```python
from build123d import *

# Parameters (mm, degrees)
EXTRUDE_2_DEPTH     = 6
SKETCH_2_R          = 1.55
CUT_EXTRUDE_1_DEPTH = 10
SKETCH_3_R          = 1.55
CUT_EXTRUDE_2_DEPTH = 10
EXTRUDE_4_DEPTH     = 1.5
EXTRUDE_5_DEPTH     = 1.5
SKETCH_5_W          = 6
SKETCH_5_H          = 6
EXTRUDE_6_DEPTH     = 60
CUT_EXTRUDE_3_DEPTH = 60
SKETCH_9_W          = 6
SKETCH_9_H          = 8.845903007
EXTRUDE_7_DEPTH     = 60
SKETCH_10_W         = 5
SKETCH_10_H         = 2
CUT_EXTRUDE_4_DEPTH = 10
SKETCH_11_R         = 1.55
CUT_EXTRUDE_5_DEPTH = 10


with BuildPart() as part:
    # 草图1 → 凸台-拉伸2 (new body)
    with BuildSketch(Plane(origin=(0, 0, 0), x_dir=(1, 0, 0), z_dir=(0, 1, 0))):
        Polygon((-72.757575758, -68.484848485), (-72.757575758, -1.484848485), (71.242424242, -1.484848485), (71.242424242, -68.484848485), (74.242424242, -68.484848485), (74.242424242, -1.484848485), (74.242424242, 1.515151515), (71.242424242, 1.515151515), (-72.757575758, 1.515151515), (-75.757575758, 1.515151515), (-75.757575758, -1.484848485), (-75.757575758, -68.484848485), align=None)
    extrude(amount=EXTRUDE_2_DEPTH)

    # 草图2 → 切除-拉伸1 (cut)
    with BuildSketch(Plane(origin=(-72.757575758, 0, 0), x_dir=(0, 0, -1), z_dir=(1, 0, 0))):
        with Locations((-65.484848485, 3)):
            Circle(SKETCH_2_R)
    extrude(amount=-CUT_EXTRUDE_1_DEPTH, mode=Mode.SUBTRACT)

    # 草图3 → 切除-拉伸2 (cut)
    with BuildSketch(Plane(origin=(74.242424242, 0, 0), x_dir=(0, 0, -1), z_dir=(1, 0, 0))):
        with Locations((-65.484848485, 3)):
            Circle(SKETCH_3_R)
    extrude(amount=-CUT_EXTRUDE_2_DEPTH, mode=Mode.SUBTRACT)

    # 草图6 → 凸台-拉伸4 (add)
    with BuildSketch(Plane(origin=(0, 6, 0), x_dir=(1, 0, 0), z_dir=(0, 1, 0))):
        Polygon((-75.757575758, 1.515151515), (74.242424242, 1.515151515), (74.242424242, -68.484848485), (71.242424242, -68.484848485), (71.242424242, -1.484848485), (-72.757575758, -1.484848485), (-72.757575758, -68.484848485), (-75.757575758, -68.484848485), align=None)
    extrude(amount=EXTRUDE_4_DEPTH)

    # 草图7 → 凸台-拉伸5 (add)
    with BuildSketch(Plane.XZ):
        Polygon((-75.757575758, 68.484848485), (-75.757575758, -1.515151515), (74.242424242, -1.515151515), (74.242424242, 68.484848485), (71.242424242, 68.484848485), (71.242424242, 1.484848485), (-72.757575758, 1.484848485), (-72.757575758, 68.484848485), align=None)
    extrude(amount=EXTRUDE_5_DEPTH)

    # 草图5 → 凸台-拉伸6 (add)
    with BuildSketch(Plane(origin=(0, 0, -1.515151515), x_dir=(-1, 0, 0), z_dir=(0, 0, -1))):
        with Locations((0.757575758, 3)):
            Rectangle(SKETCH_5_W, SKETCH_5_H)
    extrude(amount=EXTRUDE_6_DEPTH)

    # 草图8 → 切除-拉伸3 (cut)
    with BuildSketch(Plane(origin=(2.242424242, 0, 0), x_dir=(0, 0, -1), z_dir=(1, 0, 0))):
        Polygon((61.515151515, 6), (55.015151515, 0), (61.515151515, 0), align=None)
    extrude(amount=-CUT_EXTRUDE_3_DEPTH, mode=Mode.SUBTRACT)

    # 草图9 → 凸台-拉伸7 (add)
    with BuildSketch(Plane(origin=(0, -27.419692129, -25.310485042), x_dir=(1, 0, 0), z_dir=(0, -0.7348034446274878, -0.678280102733066))):
        with Locations((-0.757575758, -44.848274344)):
            Rectangle(SKETCH_9_W, SKETCH_9_H)
    extrude(amount=EXTRUDE_7_DEPTH)

    # 草图10 → 切除-拉伸4 (cut)
    with BuildSketch(Plane(origin=(0, -71.507898807, -66.007291206), x_dir=(1, 0, 0), z_dir=(0, -0.7348034446274876, -0.6782801027330662))):
        with Locations((-0.757575758, -44.848274343)):
            Rectangle(SKETCH_10_W, SKETCH_10_H)
    extrude(amount=-CUT_EXTRUDE_4_DEPTH, mode=Mode.SUBTRACT)

    # 草图11 → 切除-拉伸5 (cut)
    with BuildSketch(Plane(origin=(0, 33.419692129, -36.204666473), x_dir=(-1, 0, 0), z_dir=(0, 0.6782801027330662, -0.7348034446274876))):
        with Locations(Location((0.757575758, -90.315682622, 0), (0, 0, 90))):
            Circle(SKETCH_11_R)
    extrude(amount=-CUT_EXTRUDE_5_DEPTH, mode=Mode.SUBTRACT)


solid = part.part
```
Could you check a few things on this model? Use its own coordinates, in mm. A direction names the side the tool comes from. Round coordinates to 2 decimals unless told otherwise and drop trailing zeros. Loops run counter-clockwise (first coordinate to the right, second up) from the corner with the lowest first, then second, coordinate; pieces in that order, holes last. Notation, with made-up numbers: (56.25, 60) - (64.25, 60) arc R16 cw to (64.25, 83) - close; hole circle Ø2 at (-8.5, 42). An arc over 180 degrees is marked (long way). Answer as CSV lines item,"result".
1. I want a section at C-C on z = -36. List the corners of the cut face in (x, y) for me, then the cut area to 3 significant figures.
Filled in:
outline,"(-3.76, 0) - (2.24, 0) - (2.24, 6) - (-3.76, 6) - close"
area,"36.0 mm^2"
2. On a 3-axis mill with a long thin cutter (end or side, diameter ignored), from which of +Z, -Z, +X, -X, +Y, -Y can I reach the whole of each face in a straight line? I mean faces 1 (the face through (-0.79, -38.14, -94.88)), 2 (the face through (71.242, 3, 35)), 3 (the face through (2.242, -9, -65)), 4 (the face through (-1, 6, -31)). Say none if no direction works.
Filled in:
face 1,"none"
face 2,"+Z, +Y, -Y"
face 3,"-Z, +X, +Y, -Y"
face 4,"-Z, +X, -X, +Y"
3. We'd pull the mould along X, two halves only. Please class faces 5 (the face through (-3.758, -9, -65)), 6 (the face through (-0.8, -15.735, -81.579)), 7 (the face through (1.742, -37, -96)), 8 (the face through (-0.793, -36.787, -96.353)): +X half, -X half, draft (parallel to the pull), parting line (faces both ways), or undercut.
Filled in:
face 5,"-X half"
face 6,"draft"
face 7,"undercut"
face 8,"undercut"
4. Please list where these lines run through material, in increasing order: line 1 along Z through (x, y) = (-46, 3); line 2 along X through (y, z) = (-0.5, 16); line 3 along X through (y, z) = (4.5, -21.5). Write a range as [from, to].
Filled in:
line 1,"z = [-1.52, 1.48]"
line 2,"x = [-75.76, -72.76], [71.24, 74.24]"
line 3,"x = [-3.76, 2.24]"
5. I want a section at A-A on z = 22.5. List the corners of the cut face in (x, y) for me, then the cut area to 3 significant figures.
Filled in:
outline,"(-75.76, -1.5) - (-72.76, -1.5) - (-72.76, 7.5) - (-75.76, 7.5) - close; (71.24, -1.5) - (74.24, -1.5) - (74.24, 7.5) - (71.24, 7.5) - close"
area,"54.0 mm^2"
6. For pin 1 Ø9 at (y, z) = (-39.5, -94) entering from -X; pin 2 Ø2.5 at (y, z) = (3, 65.48) entering from -X; pin 3 Ø9 at (y, z) = (-38, -97.5) entering from +X; pin 4 Ø5 at (x, z) = (0.5, -45.5) entering from +Y, each with a flat end and sliding along its axis, tell me the tip position at first contact or that it passes through.
Filled in:
pin 1,"stops at x = -3.76"
pin 2,"passes through"
pin 3,"stops at x = 2.24"
pin 4,"stops at y = 6"
7. I want a section at B-B on x = 65. List the corners of the cut face in (y, z) for me.
Filled in:
outline,"(-1.5, -1.52) - (7.5, -1.52) - (7.5, 1.48) - (-1.5, 1.48) - close"
